Source: CAD feature listing. Evaluate the final solid. Frame: model axes, mm. Face numbers are marked on the shaded views. A direction names the side the tool comes from. Round coordinates to 2 decimals unless told otherwise and drop trailing zeros. Write each loop counter-clockwise with the first axis right and the second up, starting at its lowest first coordinate (ties: lowest second). Pieces come first, ordered by that corner, then holes. Notation, with made-up numbers: M 66,-7.75 L 111,-7.75 A21 ccw 111,20.25 Z; hole C 86.25,-10 d2. An arc over 180 degrees is marked long. Use a Markdown table: item, result.
```python
from build123d import *

# Parameters (mm, degrees)
CYLINDER005_R             = 3
CYLINDER005_DEPTH         = 10
BOX009_W                  = 30
BOX009_H                  = 30
BOX009_DEPTH              = 6
FUSION005_PLACEMENT_ANGLE = 270
BOX008_W                  = 28
BOX008_H                  = 18
BOX008_DEPTH              = 12.2
BOX007_W                  = 10
BOX007_H                  = 10
BOX007_DEPTH              = 10
BOX006_W                  = 10
BOX006_H                  = 10
BOX006_DEPTH              = 10
BOX005_W                  = 10
BOX005_H                  = 8
BOX005_DEPTH              = 4
BOX004_W                  = 29
BOX004_H                  = 19.5
BOX004_DEPTH              = 7.25
CYLINDER004_R             = 3.6
CYLINDER004_DEPTH         = 6.7
CYLINDER003_R             = 4.65
CYLINDER003_DEPTH         = 19
CYLINDER002_R             = 3.6
CYLINDER002_DEPTH         = 6.7
CYLINDER001_R             = 4.65
CYLINDER001_DEPTH         = 19
BOX003_W                  = 50
BOX003_H                  = 27
BOX003_DEPTH              = 12
BOX002_W                  = 51
BOX002_H                  = 24
BOX002_DEPTH              = 7
BOX001_W                  = 51
BOX001_H                  = 28
BOX001_DEPTH              = 6
FUSION001_PLACEMENT_ANGLE = 90
CYLINDER_R                = 6.5
CYLINDER_DEPTH            = 9
BOX_W                     = 30
BOX_H                     = 16
BOX_DEPTH                 = 30
FUSION_PLACEMENT_ANGLE    = 90
BOX013_W                  = 27
BOX013_H                  = 15.5
BOX013_DEPTH              = 3.5
BOX012_W                  = 75
BOX012_H                  = 64
BOX012_DEPTH              = 4
BOX011_W                  = 67
BOX011_H                  = 56
BOX011_DEPTH              = 30
BOX010_W                  = 75
BOX010_H                  = 64
BOX010_DEPTH              = 36
FILLET_R                  = 1.5


with BuildPart() as cylinder005:
    # Cylinder005 → Cylinder005 (new body)
    with BuildSketch(Plane(origin=(15, 15, 0), x_dir=(1, 0, 0), z_dir=(0, 0, 1))):
        Circle(CYLINDER005_R)
    extrude(amount=CYLINDER005_DEPTH)


with BuildPart() as obj1:
    # Box009 → Box009 (new body)
    with BuildSketch(Plane.XY):
        with Locations((15, 15)):
            Rectangle(BOX009_W, BOX009_H)
    extrude(amount=BOX009_DEPTH)

    # Fusion005: union Cylinder005
    add(cylinder005.part)


with BuildPart() as obj1_1:
    # Fusion005 placement: moved
    add(obj1.part.moved(Location((-34, 0, 0))).rotate(Axis((-34, 0, 0), (0, 1, 0)), FUSION005_PLACEMENT_ANGLE))


with BuildPart() as obj2:
    # Box008 → Box008 (new body)
    with BuildSketch(Plane(origin=(-30, -7, 0), x_dir=(1, 0, 0), z_dir=(0, 0, 1))):
        with Locations((14, 9)):
            Rectangle(BOX008_W, BOX008_H)
    extrude(amount=BOX008_DEPTH)


with BuildPart() as cube006:
    # Box007 → Box007 (new body)
    with BuildSketch(Plane(origin=(19, 14.5, 4), x_dir=(1, 0, 0), z_dir=(0, 0, 1))):
        with Locations((5, 5)):
            Rectangle(BOX007_W, BOX007_H)
    extrude(amount=BOX007_DEPTH)


with BuildPart() as cube005:
    # Box006 → Box006 (new body)
    with BuildSketch(Plane(origin=(19, -5, 4), x_dir=(1, 0, 0), z_dir=(0, 0, 1))):
        with Locations((5, 5)):
            Rectangle(BOX006_W, BOX006_H)
    extrude(amount=BOX006_DEPTH)


with BuildPart() as cube004:
    # Box005 → Box005 (new body)
    with BuildSketch(Plane(origin=(28, 5.75, 1.75), x_dir=(1, 0, 0), z_dir=(0, 0, 1))):
        with Locations((5, 4)):
            Rectangle(BOX005_W, BOX005_H)
    extrude(amount=BOX005_DEPTH)


with BuildPart() as usb_battery_charger:
    # Box004 → Box004 (new body)
    with BuildSketch(Plane.XY):
        with Locations((14.5, 9.75)):
            Rectangle(BOX004_W, BOX004_H)
    extrude(amount=BOX004_DEPTH)

    # Fusion004: union Cube004
    add(cube004.part)

    # Cut: cut Cube005
    add(cube005.part, mode=Mode.SUBTRACT)

    # Cut001: cut Cube006
    add(cube006.part, mode=Mode.SUBTRACT)


with BuildPart() as usb_battery_charger_1:
    # Cut001 placement: moved
    add(usb_battery_charger.part.moved(Location((4, -8, 0))))


with BuildPart() as cylinder004:
    # Cylinder004 → Cylinder004 (new body)
    with BuildSketch(Plane.XY.offset(19)):
        Circle(CYLINDER004_R)
    extrude(amount=CYLINDER004_DEPTH)


with BuildPart() as push_button_start_stop:
    # Cylinder003 → Cylinder003 (new body)
    with BuildSketch(Plane.XY):
        Circle(CYLINDER003_R)
    extrude(amount=CYLINDER003_DEPTH)

    # Fusion003: union Cylinder004
    add(cylinder004.part)


with BuildPart() as push_button_start_stop_1:
    # Fusion003 placement: moved
    add(push_button_start_stop.part.moved(Location((3, 35, 12))))


with BuildPart() as cylinder002:
    # Cylinder002 → Cylinder002 (new body)
    with BuildSketch(Plane.XY.offset(19)):
        Circle(CYLINDER002_R)
    extrude(amount=CYLINDER002_DEPTH)


with BuildPart() as push_button_mode_reset:
    # Cylinder001 → Cylinder001 (new body)
    with BuildSketch(Plane.XY):
        Circle(CYLINDER001_R)
    extrude(amount=CYLINDER001_DEPTH)

    # Fusion002: union Cylinder002
    add(cylinder002.part)


with BuildPart() as push_button_mode_reset_1:
    # Fusion002 placement: moved
    add(push_button_mode_reset.part.moved(Location((20, 35, 12))))


with BuildPart() as lipo_battery:
    # Box003 → Box003 (new body)
    with BuildSketch(Plane(origin=(-22, 18, 0), x_dir=(1, 0, 0), z_dir=(0, 0, 1))):
        with Locations((25, 13.5)):
            Rectangle(BOX003_W, BOX003_H)
    extrude(amount=BOX003_DEPTH)


with BuildPart() as cube002:
    # Box002 → Box002 (new body)
    with BuildSketch(Plane(origin=(0, 2, 6), x_dir=(1, 0, 0), z_dir=(0, 0, 1))):
        with Locations((25.5, 12)):
            Rectangle(BOX002_W, BOX002_H)
    extrude(amount=BOX002_DEPTH)


with BuildPart() as lcd_display:
    # Box001 → Box001 (new body)
    with BuildSketch(Plane.XY):
        with Locations((25.5, 14)):
            Rectangle(BOX001_W, BOX001_H)
    extrude(amount=BOX001_DEPTH)

    # Fusion001: union Cube002
    add(cube002.part)


with BuildPart() as lcd_display_1:
    # Fusion001 placement: moved
    add(lcd_display.part.moved(Location((-5, -8, 25))).rotate(Axis((-5, -8, 25), (0, 0, 1)), FUSION001_PLACEMENT_ANGLE))


with BuildPart() as cylinder:
    # Cylinder → Cylinder (new body)
    with BuildSketch(Plane(origin=(15, 8, 30), x_dir=(1, 0, 0), z_dir=(0, 0, 1))):
        Circle(CYLINDER_R)
    extrude(amount=CYLINDER_DEPTH)


with BuildPart() as awesome_switch:
    # Box → Box (new body)
    with BuildSketch(Plane.XY):
        with Locations((15, 8)):
            Rectangle(BOX_W, BOX_H)
    extrude(amount=BOX_DEPTH)

    # Fusion: union Cylinder
    add(cylinder.part)


with BuildPart() as awesome_switch_1:
    # Fusion placement: moved
    add(awesome_switch.part.moved(Location((-11, 17, 8))).rotate(Axis((-11, 17, 8), (1, 0, 0)), FUSION_PLACEMENT_ANGLE))


with BuildPart() as parts:
    # Box013 → Box013 (new body)
    with BuildSketch(Plane(origin=(-35, 19, 12), x_dir=(1, 0, 0), z_dir=(0, 0, 1))):
        with Locations((13.5, 7.75)):
            Rectangle(BOX013_W, BOX013_H)
    extrude(amount=BOX013_DEPTH)

    # Fusion006: union obj1, obj2, USB Battery Charger, Push Button start/stop, Push Button mode/reset, Lipo Battery, LCD Display, Awesome switch
    add(obj1_1.part)
    add(obj2.part)
    add(usb_battery_charger_1.part)
    add(push_button_start_stop_1.part)
    add(push_button_mode_reset_1.part)
    add(lipo_battery.part)
    add(lcd_display_1.part)
    add(awesome_switch_1.part)


with BuildPart() as lidremove:
    # Box012 → Box012 (new body)
    with BuildSketch(Plane(origin=(-42, -15, 30), x_dir=(1, 0, 0), z_dir=(0, 0, 1))):
        with Locations((37.5, 32)):
            Rectangle(BOX012_W, BOX012_H)
    extrude(amount=BOX012_DEPTH)


with BuildPart() as innerbox:
    # Box011 → Box011 (new body)
    with BuildSketch(Plane(origin=(-38, -11, 0), x_dir=(1, 0, 0), z_dir=(0, 0, 1))):
        with Locations((33.5, 28)):
            Rectangle(BOX011_W, BOX011_H)
    extrude(amount=BOX011_DEPTH)


with BuildPart() as cut004:
    # Box010 → Box010 (new body)
    with BuildSketch(Plane(origin=(-42, -15, -3), x_dir=(1, 0, 0), z_dir=(0, 0, 1))):
        with Locations((37.5, 32)):
            Rectangle(BOX010_W, BOX010_H)
    extrude(amount=BOX010_DEPTH)

    # Fillet
    fillet_edges = [cut004.edges().sort_by_distance(p)[0] for p in [
        (-42, -15, 15),
        (-42, 17, 33),
        (-42, 49, 15),
        (-42, 17, -3),
        (33, -15, 15),
        (33, 17, 33),
        (33, 49, 15),
        (33, 17, -3),
        (-4.5, -15, -3),
        (-4.5, -15, 33),
        (-4.5, 49, -3),
        (-4.5, 49, 33),
    ]]
    fillet(fillet_edges, radius=FILLET_R)

    # Cut002: cut InnerBox
    add(innerbox.part, mode=Mode.SUBTRACT)

    # Cut003: cut LidRemove
    add(lidremove.part, mode=Mode.SUBTRACT)

    # Cut004: cut parts
    add(parts.part, mode=Mode.SUBTRACT)


solid = cut004.part
```
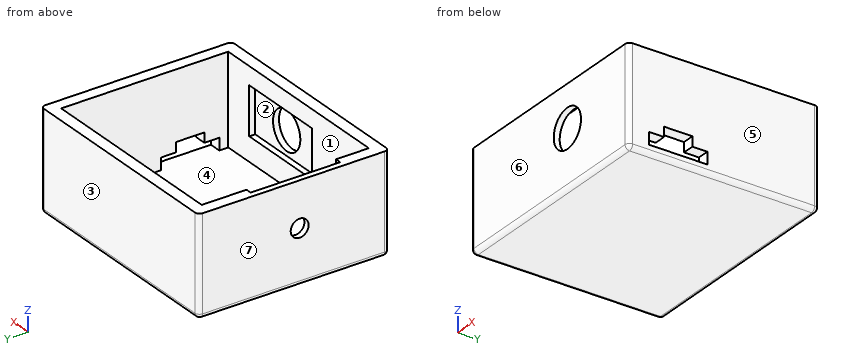
Q1. Section B-B on x = 4. Return loops of the section in (y, z), plus the area to 3 significant figures.
Results are:
| item | result |
|---|---|
| outline | M -15,-1.5 A1.5 ccw -13.5,-3 L 47.5,-3 A1.5 ccw 49,-1.5 L 49,30 L 45,30 L 45,0 L -11,0 L -11,8 L -13,8 L -13,9.5 L -15,9.5 Z; M -15,22.5 L -13,22.5 L -13,24 L -11,24 L -11,30 L -15,30 Z |
| area | 373 mm^2 |
Q2. First-contact query: pin 1 Ø10 at (y, z) = (-5, 2) entering from +X; pin 2 Ø10 at (x, y) = (18.5, -5) entering from +Z. Flat tips, straight axial feed; report the tip coordinate or a pass-through.
Results are:
| item | result |
|---|---|
| pin 1 | x = 33 |
| pin 2 | z = 0 |
Q3. Reachability of the marked faces 1, 2 and 3 from +Z, -Z, +X, -X, +Y, -Y: full face, straight path, thin tool, end or side. Return the list, or none.
Results are:
| item | result |
|---|---|
| face 1 | +Z |
| face 2 | none |
| face 3 | +Z, -Z, +X, -X, +Y |
Q4. Section D-D on y = 28. Return loops of the section in (x, z), plus the area to 3 significant figures.
Results are:
| item | result |
|---|---|
| outline | M -42,-1.5 A1.5 ccw -40.5,-3 L 31.5,-3 A1.5 ccw 33,-1.5 L 33,30 L 29,30 L 29,0 L -40,0 L -40,30 L -42,30 Z |
| area | 404 mm^2 |
Q5. Section A-A on y = 15. Return loops of the section in (x, z), plus the area to 3 significant figures.
Results are:
| item | result |
|---|---|
| outline | M -42,-1.5 A1.5 ccw -40.5,-3 L 31.5,-3 A1.5 ccw 33,-1.5 L 33,30 L 29,30 L 29,0 L -40,0 L -40,12 L -42,12 Z; M -42,18 L -40,18 L -40,30 L -42,30 Z |
| area | 392 mm^2 |
Q6. Section C-C on z = 15. Return loops of the section in (x, y).
Results are:
| item | result |
|---|---|
| outline | M -42,-13.5 A1.5 ccw -40.5,-15 L -2.42,-15 L -2.42,-13 L -11,-13 L -11,-11 L -38,-11 L -38,0 L -40,0 L -40,12 L -42,12 Z; M -42,18 L -40,18 L -40,30 L -38,30 L -38,45 L 29,45 L 29,-11 L 19,-11 L 19,-13 L 10.42,-13 L 10.42,-15 L 31.5,-15 A1.5 ccw 33,-13.5 L 33,47.5 A1.5 ccw 31.5,49 L -40.5,49 A1.5 ccw -42,47.5 Z |
Q7. Line query: L1, parallel to Y at x = 23.5, z = 7; L2, parallel to X at y = 7.5, z = 18; L3, parallel to X at y = 37.5, z = 10.5. Output: solid intervals per line, ascending.
Results are:
| item | result |
|---|---|
| L1 | -15 to -11, 45 to 49 |
| L2 | -42 to -40, 29 to 33 |
| L3 | -42 to -38, 29 to 33 |
Q8. Mould query, pull axis X, two halves, no side actions, for the marked faces 4, 5, 6 and 7. Classes: +X half, -X half, draft (parallel to the pull), parting line (faces both ways), or undercut.
Results are:
| item | result |
|---|---|
| face 4 | undercut |
| face 5 | +X half |
| face 6 | draft |
| face 7 | -X half |
